The model under review builds one solid part; all positions refer to its coordinate system, in mm. Face numbers are marked on the shaded views. A direction names the side the tool comes from. Coordinates: 2 decimals unless noted, no trailing zeros. Write each loop counter-clockwise with the first axis right and the second up, starting at its lowest first coordinate (ties: lowest second). Pieces come first, ordered by that corner, then holes.
1) For line 1 (Z direction, x = 8.75, y = 3.25); line 2 (X direction, y = 14, z = 67); line 3 (X direction, y = 13.5, z = 26), list the stretches that pass through material, from the lowest coordinate up.
2) Add section A-A, the plane x = 4.5. State the section outline as (y, z) points, then the cut area to 3 significant figures.
3) Add section B-B, the plane y = 11. State the section outline as (x, z) points (1 decimal).
4) For P1, Ø3.5, axis at x = 4.76, y = 3.84, coming from the -Z side; P2, Ø1.5, axis at x = 1.5, z = 63.5, coming from the +Y side; P3, Ø2, axis at x = 8, y = 19, coming from the +Z side; P4, Ø10, axis at y = 4.5, z = 55.5, coming from the +X side, all flat-tipped, find the tip position at first contact; note any pin that passes through.
5) Machinability: for the marked faces 1 and 2, which of the approach directions +Z, -Z, +X, -X, +Y, -Y give a long, thin tool a straight path to every point of the face, cutting with its end or side? Answer none if there is none.
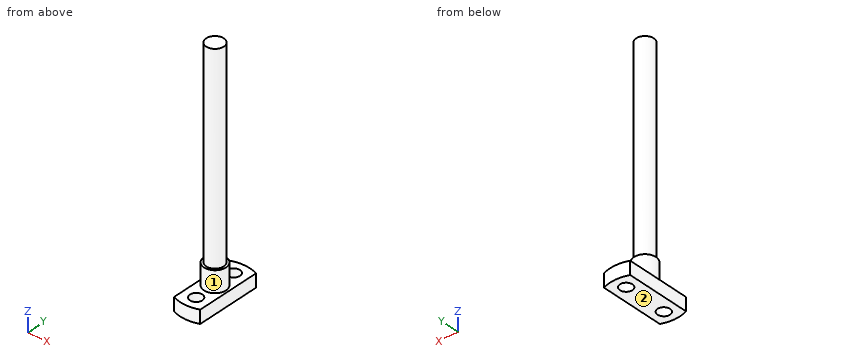
from build123d import *

# Parameters (mm, degrees)
BOSS_EXTRUDE1_DEPTH         = 4.7625
SKETCH2_R                   = 3.96875
BOSS_EXTRUDE2_DEPTH         = 7.62
SKETCH3_R                   = 3.175
BOSS_EXTRUDE3_DEPTH         = 73.025
F_16_0_177_DIAMETER_HOLE1_D = 4.4958


with BuildPart() as part:
    # Sketch1 → Boss-Extrude1 (new body)
    with BuildSketch(Plane.XY):
        with BuildLine():
            Line((0, 0), (0, 23.546430197))
            ThreePointArc((0, 23.546430197), (4.7625, 24.473215098), (9.525, 23.546430197))
            Line((9.525, 23.546430197), (9.525, 0))
            ThreePointArc((9.525, 0), (4.7625, -0.926784902), (0, 0))
        make_face()
    extrude(amount=BOSS_EXTRUDE1_DEPTH)

    # Sketch2 → Boss-Extrude2 (add)
    with BuildSketch(Plane.XY.offset(4.7625)):
        with Locations(Location((4.7625, 11.773215098, 0), (0, 0, 180))):
            Circle(SKETCH2_R)
    extrude(amount=BOSS_EXTRUDE2_DEPTH)

    # Sketch3 → Boss-Extrude3 (add)
    with BuildSketch(Plane.XY.offset(12.3825)):
        with Locations((4.7625, 11.773215098)):
            Circle(SKETCH3_R)
    extrude(amount=BOSS_EXTRUDE3_DEPTH)

    # #16 (0.177) Diameter Hole1 (through all)
    with Locations(Plane.XY.offset(4.7625)):
        with Locations((4.7625, 3.835715098), (4.7625, 19.710715098)):
            Hole(F_16_0_177_DIAMETER_HOLE1_D / 2)


solid = part.part
Geometry results:
1. line 1: z = 0 to 4.76
1. line 2: x = 2.5 to 7.03
1. line 3: x = 2.1 to 7.43
2. outline: (-0.92, 0) - (1.6, 0) - (1.6, 4.76) - (-0.92, 4.76) - close; (6.07, 0) - (17.48, 0) - (17.48, 4.76) - (15.73, 4.76) - (15.73, 12.38) - (14.94, 12.38) - (14.94, 85.41) - (8.61, 85.41) - (8.61, 12.38) - (7.81, 12.38) - (7.81, 4.76) - (6.07, 4.76) - close; (21.94, 0) - (24.47, 0) - (24.47, 4.76) - (21.94, 4.76) - close
2. area: 601 mm2
3. outline: (0, 0) - (9.5, 0) - (9.5, 4.8) - (8.7, 4.8) - (8.7, 12.4) - (7.8, 12.4) - (7.8, 85.4) - (1.7, 85.4) - (1.7, 12.4) - (0.9, 12.4) - (0.9, 4.8) - (0, 4.8) - close
4. P1: passes through
4. P2: stops at y = 13.71
4. P3: stops at z = 4.76
4. P4: stops at x = 6.98
5. face 1: +Z
5. face 2: -Z, +X, -X, +Y, -Y
